```python
from build123d import *

# Parameters (mm, degrees)
SKETCH1_W                                        = 31.75
SKETCH1_H                                        = 101.6
BOSS_EXTRUDE1_DEPTH                              = 15.875
CUT_EXTRUDE1_REACH                               = 106.051
F_1_4_20_TAPPED_HOLE1_D                          = 5.1054
CBORE_FOR_1_4_SOCKET_HEAD_CAP_SCREW1_D           = 6.7564
CBORE_FOR_1_4_SOCKET_HEAD_CAP_SCREW1_CBORE_D     = 11.1125
CBORE_FOR_1_4_SOCKET_HEAD_CAP_SCREW1_CBORE_DEPTH = 20.32


with BuildPart() as part:
    # Sketch1 → Boss-Extrude1 (new, symmetric)
    with BuildSketch(Plane(origin=(0, 0, 0), x_dir=(1, 0, 0), z_dir=(0, 1, 0))):
        Rectangle(SKETCH1_W, SKETCH1_H)
    extrude(amount=BOSS_EXTRUDE1_DEPTH, both=True)

    # Sketch2 → Cut-Extrude1 (cut, up to next)
    with BuildSketch(Plane.XY.offset(50.8), mode=Mode.PRIVATE) as cut_extrude1_sk1:
        Polygon((-15.875, -3.175), (-15.875, 15.875), (3.175, 15.875), align=None)
    cut_extrude1_tool1 = extrude(cut_extrude1_sk1.sketch, amount=-CUT_EXTRUDE1_REACH, mode=Mode.PRIVATE) & part.part
    add(cut_extrude1_tool1.solids().sort_by_distance((-9.525, 9.525, 50.8))[0], mode=Mode.SUBTRACT)

    # 1/4-20 Tapped Hole1 (through all)
    with Locations(Plane(origin=(-6.35, 6.35, 0), x_dir=(0, 0, 1), z_dir=(-0.7071067811865513, 0.7071067811865438, 0))):
        with Locations((-25.4, 0), (25.4, 0)):
            Hole(F_1_4_20_TAPPED_HOLE1_D / 2)

    # CBORE for 1/4 Socket Head Cap Screw1 (through all)
    with Locations(Plane.ZY.offset(15.875)):
        with Locations((-38.1, 3.175), (38.1, 3.175)):
            CounterBoreHole(CBORE_FOR_1_4_SOCKET_HEAD_CAP_SCREW1_D / 2, CBORE_FOR_1_4_SOCKET_HEAD_CAP_SCREW1_CBORE_D / 2, CBORE_FOR_1_4_SOCKET_HEAD_CAP_SCREW1_CBORE_DEPTH)


solid = part.part
```
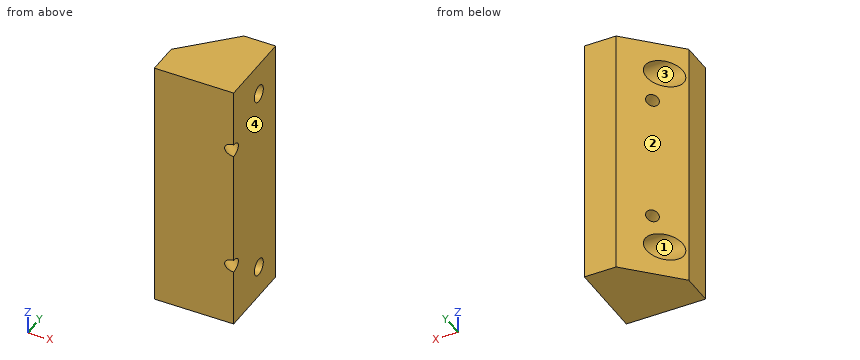
Could you check a few things on this model? Use its own coordinates, in mm. Face numbers are marked on the shaded views. Give positions to 0.01 mm unless a question says otherwise; leave off trailing zeros. Loops run counter-clockwise (first coordinate to the right, second up) from the corner with the lowest first, then second, coordinate; pieces in that order, holes last. Notation, with made-up numbers: (3.25, -28) -> (33.25, -28) arc R35 cw to (33.25, 9) -> close; hole circle Ø6 at (50.25, 72.5). An arc over 180 degrees is marked (long way). Put each result on its own line as item: value.
(1) Imagine slicing it at B-B on x = -2. State how many separate pieces and enclosed holes the cut face has, plus the area to 3 significant figures.
Computed:
separate pieces: 1
enclosed holes: 4
area: 2,450 mm^2
(2) Please list where these lines run through material, in increasing order: probe 1 along Z at (x, y) = (-11, 1); probe 2 along Z at (x, y) = (5.5, -3.5); probe 3 along Z at (x, y) = (-3.5, 6). Write a range as [from, to].
Computed:
probe 1: [-50.8, -43.21], [-32.99, 32.99], [43.21, 50.8]
probe 2: [-50.8, -27.53], [-23.27, 23.27], [27.53, 50.8]
probe 3: [-50.8, -42.88], [-33.32, -27.24], [-23.56, 23.56], [27.24, 33.32], [42.88, 50.8]
(3) Thinking about a two-plate mould opening in Y: for the marked faces 1, 2, 3 and 4, which applies, pulls with the +Y half, pulls with the -Y half, needs draft (parallel to the pull), parting line crosses it, or undercut?
Computed:
face 1: undercut
face 2: pulls with the +Y half
face 3: undercut
face 4: needs draft
(4) Imagine slicing it at C-C on z = -13. Write out the boundary of the cut face in (x, y) (3 decimals).
Computed:
outline: (-15.875, -15.875) -> (15.875, -15.875) -> (15.875, 15.875) -> (3.175, 15.875) -> (-15.875, -3.175) -> close
(5) I'm going to push flat-ended pins straight in: pin 1 Ø12 at (y, z) = (3.5, -36.5) entering from -X; pin 2 Ø18 at (y, z) = (3.175, -38.1) entering from -X (3 decimals); pin 3 Ø10 at (y, z) = (3.175, 38.1) entering from -X (3 decimals); pin 4 Ø12 at (x, z) = (-4.5, -21.5) entering from +Y. Where does each tip first touch, or does it pass through?
Computed:
pin 1: x = -15.2
pin 2: x = -15.875
pin 3: x = 4.445
pin 4: y = 14.2
(6) Imagine slicing it at A-A on z = -38.1. Write out the boundary of the cut face in (x, y) (3 decimals).
Computed:
outline: (-15.875, -15.875) -> (15.875, -15.875) -> (15.875, -0.203) -> (4.445, -0.203) -> (4.445, -2.381) -> (-15.081, -2.381) -> (-15.875, -3.175) -> close; (-3.969, 8.731) -> (4.445, 8.731) -> (4.445, 6.553) -> (15.875, 6.553) -> (15.875, 15.875) -> (3.175, 15.875) -> close
